Verification items for the finished model (mm, model axes). A direction names the side the tool comes from. Give positions to 0.01 mm unless a question says otherwise; leave off trailing zeros. Write each loop counter-clockwise with the first axis right and the second up, starting at its lowest first coordinate (ties: lowest second). Pieces come first, ordered by that corner, then holes. Notation, with made-up numbers: (-2.75, 3) -> (35.25, 3) arc R23 cw to (35.25, 28) -> close; hole circle Ø1 at (-16.75, 69.5). An arc over 180 degrees is marked (long way). Answer as CSV lines item,"result".
```python
from build123d import *

# Parameters (mm, degrees)
F0_W     = 10.16
F0_H     = 130.5052
F1_DEPTH = 38.1
F5_DEPTH = 25.4
F3_W     = 5.2832
F3_H     = 25.4
F6_DEPTH = 152.4


with BuildPart() as f1:
    # F0 (on Front) → F1 (new body)
    with BuildSketch(Plane.XZ):
        with Locations((9.568245, -12.447174)):
            Rectangle(F0_W, F0_H)
    extrude(amount=F1_DEPTH)

    # F4 (on face) → F5 (cut)
    with BuildSketch(Plane(origin=(4.488245, 0, 0), x_dir=(0, -1, 0), z_dir=(-1, 0, 0))):
        with BuildLine():
            Line((0, 36.306467), (0, -53.210054))
            ThreePointArc((0, -53.210054), (4.081656, -8.451793), (0, 36.306467))
        make_face()
    extrude(amount=-F5_DEPTH, mode=Mode.SUBTRACT)

    # F3 (on face) → F6 (cut)
    with BuildSketch(Plane.XY.offset(52.805426)):
        with Locations((9.568245, -19.05)):
            Rectangle(F3_W, F3_H)
    extrude(amount=-F6_DEPTH, mode=Mode.SUBTRACT)


solid = f1.part
```
1) Tool access check on faces 4 (the flat face through (10, -31.75, -12)), 5 (the flat face through (6, -19, -77.7)). Record the directions out of +Z, -Z, +X, -X, +Y, -Y that give a thin tool (end or side, any length) a straight path to the whole face; none if there is none.
Reported:
face 4,"+Z, -Z"
face 5,"-Z, +X, -X, +Y, -Y"
2) Section check B-B (x = 9.5). Record the boundary of the cut face in (y, z).
Reported:
outline,"(-38.1, -77.7) -> (-31.75, -77.7) -> (-31.75, 52.81) -> (-38.1, 52.81) -> close; (-6.35, -77.7) -> (0, -77.7) -> (0, -53.21) arc R247.44 cw to (0, 36.31) -> (0, 52.81) -> (-6.35, 52.81) -> close"
3) Scan lines: line 1 along X through (y, z) = (-15.5, -17.5); line 2 along Y through (x, z) = (11, -10); line 3 along Y through (x, z) = (11.75, -57.5). Record each from-to range of solid material in increasing order.
Reported:
line 1,"4.49 to 6.93, 12.21 to 14.65"
line 2,"-38.1 to -31.75, -6.35 to -4.08"
line 3,"-38.1 to -31.75, -6.35 to 0"
4) Draft check along X on faces 1 (the cylindrical face through (9.5, -4.08, -9.08)), 2 (the flat face through (4.488, -19, -13)), 3 (the flat face through (12.21, -19, -12)). Enter one of: +X half, -X half, draft (parallel to the pull), parting line (faces both ways), or undercut.
Reported:
face 1,"draft"
face 2,"-X half"
face 3,"undercut"
5) Depth check by flat-ended pin: pin 1 (4 mm diameter, centred on x = 12, z = 22, fed in from +Y); pin 2 (2.5 mm diameter, centred on x = 10.5, z = -27.5, fed in from +Y); pin 3 (2 mm diameter, centred on x = 7, z = -26, fed in from +Y). Enter the tip coordinate at first touch or a pass-through.
Reported:
pin 1,"y = -1.94"
pin 2,"y = -3.25"
pin 3,"y = -3.39"
6) Section check A-A (y = -17). Record the boundary of the cut face in (x, z).
Reported:
outline,"(4.49, -77.7) -> (6.93, -77.7) -> (6.93, 52.81) -> (4.49, 52.81) -> close; (12.21, -77.7) -> (14.65, -77.7) -> (14.65, 52.81) -> (12.21, 52.81) -> close"
7) Section check C-C (z = -13.5). Record the boundary of the cut face in (x, y).
Reported:
outline,"(4.49, -38.1) -> (14.65, -38.1) -> (14.65, -4.03) -> (4.49, -4.03) -> close; hole (6.93, -31.75) -> (12.21, -31.75) -> (12.21, -6.35) -> (6.93, -6.35) -> close"
8) Section check D-D (z = -62). Record the boundary of the cut face in (x, y).
Reported:
outline,"(4.49, -38.1) -> (14.65, -38.1) -> (14.65, 0) -> (4.49, 0) -> close; hole (6.93, -31.75) -> (12.21, -31.75) -> (12.21, -6.35) -> (6.93, -6.35) -> close"
